Drawing for the job (mm, zero at the part's lowest x, y, z). A direction names the side the tool comes from. Give positions to 0.01 mm unless a question says otherwise; leave off trailing zeros. Order: outer loops, then holes, each group sorted by start corner. A loop starts at its lowest first (then second) coordinate and runs counter-clockwise, first axis right, second up. Notation, with made-up numbers: (80, 27) - (94, 27) arc R29 cw to (94, 54) - close; hole circle Ø11 at (-24, -19.5). An arc over 180 degrees is marked (long way). One line per item, written item: value.
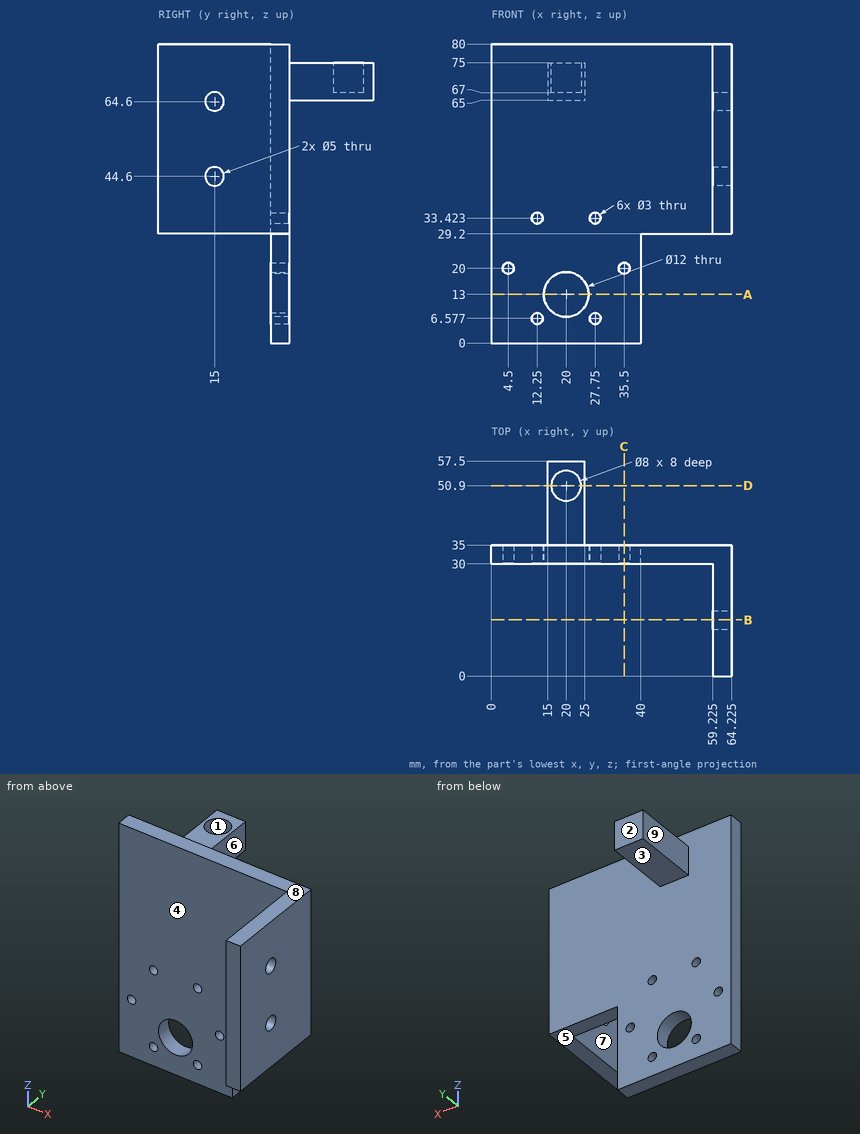
1) Cut at D-D, the plane y = 50.9. Give the cut face in (x, z), then the cut area to 3 significant figures.
Outcome:
outline: (15, 65) - (25, 65) - (25, 75) - (24, 75) - (24, 67) - (16, 67) - (16, 75) - (15, 75) - close
area: 36.0 mm^2
2) Cut at A-A, the plane z = 13. Give the cut face in (x, y).
Outcome:
outline: (0, 30) - (14, 30) - (14, 35) - (0, 35) - close; (26, 30) - (40, 30) - (40, 35) - (26, 35) - close
3) Mould opens along Y. For the marked faces 1, 2, 3 and 4 say: released by +Y, released by -Y, zero draft, split by the parting line, or undercut.
Outcome:
face 1: undercut
face 2: released by +Y
face 3: zero draft
face 4: released by -Y
4) Drill centre lines: line 1 along X through (y, z) = (32.1, 20); line 2 along Y through (x, z) = (62.85, 44.6); line 3 along Z through (x, y) = (13, 34) (1 decimal). Where is each one in solid material? Low to high. Write a range as from..to.
Outcome:
line 1: x = 0..3, 6..34, 37..40
line 2: y = 0..12.5, 17.5..35
line 3: z = 0..5.3, 7.9..32.1, 34.7..80
5) Pin check, flat tips, straight feed: pin 1 (9 mm diameter, centred on x = 20, y = 50.9, fed in from +Z); pin 2 (3.5 mm diameter, centred on x = 27.75, z = 6.58, fed in from +Y); pin 3 (6 mm diameter, centred on y = 15, z = 44.6, fed in from -X) (3 decimals); pin 4 (8 mm diameter, centred on x = 51.5, y = 25.5, fed in from +Z). Stop position of each tip, or through.
Outcome:
pin 1: stops at z = 75
pin 2: stops at y = 35
pin 3: stops at x = 59.225
pin 4: passes through
6) Cut at B-B, the plane y = 15. Give the cut face in (x, z) (1 decimal).
Outcome:
outline: (59.2, 29.2) - (64.2, 29.2) - (64.2, 42.1) - (59.2, 42.1) - close; (59.2, 47.1) - (64.2, 47.1) - (64.2, 62.1) - (59.2, 62.1) - close; (59.2, 67.1) - (64.2, 67.1) - (64.2, 80) - (59.2, 80) - close
7) Which spindle directions (+Z, -Z, +X, -X, +Y, -Y) get a long thin tool onto all of the face, cutting with end or side? Do the marked faces 5, 6, 7, 8 and 9. Say none if no direction does.
Outcome:
face 5: -Z, +X, +Y, -Y
face 6: +Z, -Z, +X, +Y
face 7: +Z, -Z, -X, -Y
face 8: +Z, +X, -X, +Y, -Y
face 9: +Z, -Z, -X, +Y
8) Cut at C-C, the plane x = 35.5. Give the cut face in (y, z).
Outcome:
outline: (30, 0) - (35, 0) - (35, 18.5) - (30, 18.5) - close; (30, 21.5) - (35, 21.5) - (35, 80) - (30, 80) - close
